```python
from build123d import *

# Parameters (mm, degrees)
SKETCH8_R           = 1.5
SKETCH8_R_2         = 7
SKETCH8_R_3         = 10.95
BOSS_EXTRUDE1_DEPTH = 5
SKETCH9_W           = 10
SKETCH9_H           = 5
SKETCH9_W_2         = 5
BOSS_EXTRUDE2_DEPTH = 5
SKETCH11_R          = 7
SKETCH11_R_2        = 2
SKETCH11_W          = 10
SKETCH11_H          = 5
BOSS_EXTRUDE4_DEPTH = 5
SKETCH11_2_W        = 10
SKETCH11_2_H        = 5
CUT_EXTRUDE1_DEPTH  = 5


with BuildPart() as part:
    # Sketch8 → Boss-Extrude1 (new body)
    with BuildSketch(Plane.XY):
        with BuildLine():
            Line((-31.585962214, 30.725), (-31.585962214, -24.275))
            Line((-31.585962214, -24.275), (-21.914037786, -24.275))
            Line((-21.914037786, -24.275), (-21.914037786, -19.275))
            Line((-21.914037786, -19.275), (-23.414037786, -19.275))
            ThreePointArc((-23.414037786, -19.275), (-24.414037786, -18.275), (-23.414037786, -17.275))
            Line((-23.414037786, -17.275), (-21.914037786, -17.275))
            Line((-21.914037786, -17.275), (-21.914037786, -13.275))
            Line((-21.914037786, -13.275), (-18.914037786, -13.275))
            Line((-18.914037786, -13.275), (-18.914037786, -17.275))
            Line((-18.914037786, -17.275), (-17.414037786, -17.275))
            ThreePointArc((-17.414037786, -17.275), (-16.414037786, -18.275), (-17.414037786, -19.275))
            Line((-17.414037786, -19.275), (-18.914037786, -19.275))
            Line((-18.914037786, -19.275), (-18.914037786, -24.275))
            Line((-18.914037786, -24.275), (21.585962214, -24.275))
            Line((21.585962214, -24.275), (23.085962214, -24.275))
            Line((23.085962214, -24.275), (23.085962214, -19.275))
            Line((23.085962214, -19.275), (21.585962214, -19.275))
            ThreePointArc((21.585962214, -19.275), (20.585962214, -18.275), (21.585962214, -17.275))
            Line((21.585962214, -17.275), (23.085962214, -17.275))
            Line((23.085962214, -17.275), (23.085962214, -13.275))
            Line((23.085962214, -13.275), (26.085962214, -13.275))
            Line((26.085962214, -13.275), (26.085962214, -17.275))
            Line((26.085962214, -17.275), (27.585962214, -17.275))
            ThreePointArc((27.585962214, -17.275), (28.585962214, -18.275), (27.585962214, -19.275))
            Line((27.585962214, -19.275), (26.085962214, -19.275))
            Line((26.085962214, -19.275), (26.085962214, -24.275))
            Line((26.085962214, -24.275), (31.585962214, -24.275))
            Line((31.585962214, -24.275), (31.585962214, -9.275))
            ThreePointArc((31.585962214, -9.275), (19.870233462, 19.009271247), (-8.414037786, 30.725))
            Line((-8.414037786, 30.725), (-18.914037786, 30.725))
            Line((-18.914037786, 30.725), (-18.914037786, 25.725))
            Line((-18.914037786, 25.725), (-17.414037786, 25.725))
            ThreePointArc((-17.414037786, 25.725), (-16.414037786, 24.725), (-17.414037786, 23.725))
            Line((-17.414037786, 23.725), (-18.914037786, 23.725))
            Line((-18.914037786, 23.725), (-18.914037786, 19.725))
            Line((-18.914037786, 19.725), (-21.914037786, 19.725))
            Line((-21.914037786, 19.725), (-21.914037786, 23.725))
            Line((-21.914037786, 23.725), (-23.414037786, 23.725))
            ThreePointArc((-23.414037786, 23.725), (-24.414037786, 24.725), (-23.414037786, 25.725))
            Line((-23.414037786, 25.725), (-21.914037786, 25.725))
            Line((-21.914037786, 25.725), (-21.914037786, 30.725))
            Line((-21.914037786, 30.725), (-31.585962214, 30.725))
        make_face()
        with Locations((-8.585962214, -11.225)):
            Circle(SKETCH8_R, mode=Mode.SUBTRACT)
        with Locations((-21.085962214, 1.275)):
            Circle(SKETCH8_R, mode=Mode.SUBTRACT)
        with Locations((-8.585962214, 1.275)):
            Circle(SKETCH8_R_2, mode=Mode.SUBTRACT)
        with Locations((10.635962214, -11.325)):
            Circle(SKETCH8_R_3, mode=Mode.SUBTRACT)
        with Locations((3.914037786, 1.275)):
            Circle(SKETCH8_R, mode=Mode.SUBTRACT)
        with Locations((-8.585962214, 13.775)):
            Circle(SKETCH8_R, mode=Mode.SUBTRACT)
    extrude(amount=BOSS_EXTRUDE1_DEPTH)

    # Sketch9 → Boss-Extrude2 (add)
    with BuildSketch(Plane(origin=(0, 0, 0), x_dir=(-1, 0, 0), z_dir=(0, 0, -1))):
        with Locations((-13.085962214, -26.775)):
            Rectangle(SKETCH9_W, SKETCH9_H)
        with Locations((8.914037786, -26.775)):
            Rectangle(SKETCH9_W, SKETCH9_H)
        with BuildLine():
            Line((31.585962214, 30.725), (-31.585962214, 30.725))
            Line((-31.585962214, 30.725), (-31.585962214, 11.746641407))
            Line((-31.585962214, 11.746641407), (-31.585962214, -2.994966805))
            Line((-31.585962214, -2.994966805), (-31.585962214, -9.275))
            Line((-31.585962214, -9.275), (-26.161018226, -9.275))
            Line((-26.161018226, -9.275), (-26.161018226, -2.994966805))
            Line((-26.161018226, -2.994966805), (-17.743215339, -2.994966805))
            Line((-17.743215339, -2.994966805), (-17.743215339, 11.746641407))
            Line((-17.743215339, 11.746641407), (6.40967317, 11.746641407))
            ThreePointArc((6.40967317, 11.746641407), (8.585962214, 16.749974384), (10.762251258, 11.746641407))
            Line((10.762251258, 11.746641407), (31.585962214, 11.746641407))
            Line((31.585962214, 11.746641407), (31.585962214, 30.725))
        make_face()
        with Locations((29.085962214, -26.775)):
            Rectangle(SKETCH9_W_2, SKETCH9_H)
    extrude(amount=-BOSS_EXTRUDE2_DEPTH)

    # Sketch11 → Boss-Extrude4 (add)
    # profile 1 of 3: a face of its own
    with BuildSketch(Plane.XY.offset(5)):
        with Locations((0, 32.725)):
            Circle(SKETCH11_R)
        with Locations((0, 32.725)):
            Circle(SKETCH11_R_2, mode=Mode.SUBTRACT)
    # profile 2 of 3: a face of its own
    with BuildSketch(Plane.XY.offset(5)):
        with Locations((-16.585962214, 28.225)):
            Rectangle(SKETCH11_W, SKETCH11_H)
    # profile 3 of 3: a face of its own
    with BuildSketch(Plane.XY.offset(5)):
        with Locations((16.585962214, 28.225)):
            Rectangle(SKETCH11_W, SKETCH11_H)
    extrude(amount=-BOSS_EXTRUDE4_DEPTH)

    # Sketch11<2> → Cut-Extrude1 (cut)
    with BuildSketch(Plane.XY.offset(5)):
        with Locations((-16.585962214, 28.225)):
            Rectangle(SKETCH11_2_W, SKETCH11_2_H)
        with Locations((16.585962214, 28.225)):
            Rectangle(SKETCH11_2_W, SKETCH11_2_H)
    extrude(amount=-CUT_EXTRUDE1_DEPTH, mode=Mode.SUBTRACT)


solid = part.part
```
Source: CAD feature listing. Evaluate the final solid. Frame: model axes, mm. A direction names the side the tool comes from. Give positions to 0.01 mm unless a question says otherwise; leave off trailing zeros. Loops run counter-clockwise (first coordinate to the right, second up) from the corner with the lowest first, then second, coordinate; pieces in that order, holes last. Notation, with made-up numbers: (17, 42) - (44, 42) arc R8 cw to (44, 48) - close; hole circle Ø9 at (18, 46). An arc over 180 degrees is marked (long way). Use CSV: the item, a comma, the result in double quotes. Start each with the question number.
1. Section A-A (x = -20.5). Output: boundary loops of the cut face in (y, z) (3 decimals), then the cut area to 3 significant figures.
2. Ray query, L1, parallel to X at y = 29, z = 3.5; L2, parallel to Y at x = -23, z = 0.8 (3 decimals); L3, parallel to X at y = 0, z = 3.5. Return the intervals inside material, ascending.
3. Section C-C (z = 1.7). Count the separate pieces of the cut face and the enclosed holes in it, then the cut area to 3 significant figures.
4. Draft query along Y for faces 1 (the flat face through (-18.914, -22, 2)), 2 (the flat face through (-18, -19.275, 2)), 3 (the cylindrical face through (20.586, -18.297, 2.465)), 4 (the flat face through (29, -24.275, 2)). Return one class per face: +Y half, -Y half, draft (parallel to the pull), parting line (faces both ways), or undercut.
5. Reachability of faces 5 (the flat face through (21, -24.275, 2)), 6 (the flat face through (-18.914, -15, 2)), 7 (the flat face through (-11.586, 28, 3)), 8 (the flat face through (-27, 30.725, 2)) from +Z, -Z, +X, -X, +Y, -Y: full face, straight path, thin tool, end or side. Return the list, or none.
6. Pin query (flat end, axial travel): pin 1 (3 mm diameter, centred on x = 19.5, z = 1, fed in from +Y) (3 decimals); pin 2 (2.5 mm diameter, centred on x = 26.5, z = 2, fed in from +Y) (3 decimals); pin 3 (3 mm diameter, centred on x = -1, z = 2, fed in from -Y) (3 decimals). Return the tip coordinate at first contact, or that it passes through.
7. Section B-B (x = 9). Output: boundary loops of the cut face in (y, z) (3 decimals), then the cut area to 3 significant figures.
Response:
1,outline,"(-13.275, 0) - (-0.106, 0) - (-0.106, 5) - (-13.275, 5) - close; (2.656, 0) - (25.725, 0) - (25.725, 5) - (2.656, 5) - close"
1,area,"181 mm²"
2,L1,"-31.59 to -21.59, -11.59 to 11.59, 21.59 to 31.59"
2,L2,"-24.275 to -19.275, -17.275 to 30.725"
2,L3,"-31.59 to -21.88, -20.3 to -15.47, -1.7 to 3.12, 4.7 to 31.59"
3,separate pieces,"1"
3,enclosed holes,"7"
3,area,"2,950 mm²"
4,face 1,"draft"
4,face 2,"undercut"
4,face 3,"undercut"
4,face 4,"-Y half"
5,face 5,"+Z, -Z, +X, -Y"
5,face 6,"+Z, -Z, -Y"
5,face 7,"+Z, -Z, +Y"
5,face 8,"+Z, -Z, -X, +Y"
6,pin 1,"y = 25.725"
6,pin 2,"y = 30.725"
6,pin 3,"y = -24.275"
7,outline,"(-29.275, 0) - (-22.152, 0) - (-22.152, 5) - (-29.275, 5) - close; (-0.498, 0) - (30.725, 0) - (30.725, 5) - (-0.498, 5) - close"
7,area,"192 mm²"
